Can you work these out from the model? Positions are in its coordinate system, mm. Face numbers are marked on the shaded views. A direction names the side the tool comes from. Give positions to 0.01 mm unless a question says otherwise; leave off trailing zeros. Loops run counter-clockwise (first coordinate to the right, second up) from the corner with the lowest first, then second, coordinate; pieces in that order, holes last. Notation, with made-up numbers: (-38, 30.25) -> (-3, 30.25) arc R29 cw to (-3, 63.25) -> close; hole circle Ø4 at (32, -11). An arc over 180 degrees is marked (long way). One line per question, with ' | ' between items.
from build123d import *

# Parameters (mm, degrees)
F0_R     = 11.5
F1_DEPTH = 1.5
F3_R     = 6.1353913868
F3_R_2   = 4
F4_DEPTH = 0.762
F2_R     = 4
F5_DEPTH = 3


# Not quite as in the source:
# - a fillet or chamfer that OpenCascade refuses, or shapes differently, is made with other operations: its cross-section is extruded or revolved along the edge and cut away or added


with BuildPart() as f1:
    # F0 (on Top) → F1 (new body)
    with BuildSketch(Plane.XY):
        Circle(F0_R)
    extrude(amount=F1_DEPTH)

    # F3 (on face) → F4 (join)
    with BuildSketch(Plane.XY.offset(1.5)):
        Circle(F3_R)
        Circle(F3_R_2, mode=Mode.SUBTRACT)
    extrude(amount=F4_DEPTH)

    # F2 (on face) → F5 (join)
    with BuildSketch(Plane.XY.offset(1.5)):
        Circle(F2_R)
    extrude(amount=F5_DEPTH)

    # F6: fillet of radius 3.6792614691 on 1 edges, made by hand

    # F6_s1 → F6_t2 (revolve, cut)
    with BuildSketch(Plane.XZ):
        with BuildLine():
            ThreePointArc((11.5, 1.5), (10.1967383184, 0.396348303), (8.5355802579, 0))
            Line((8.5355802579, 0), (11.5, 0))
            Line((11.5, 0), (11.5, 1.5))
        make_face()
    revolve(axis=Axis((0, 0, 0), (0, 0, 1)), mode=Mode.SUBTRACT)


solid = f1.part
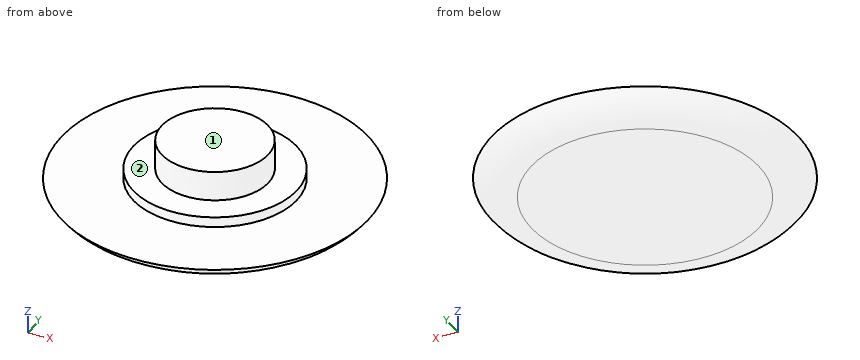
Q1. If we section it at D-D (z = 1.1): Write out the boundary of the cut face in (x, y).
Entries:
outline: circle Ø22.32 at (0, 0)
Q2. If we section it at C-C (z = 3.9): Write out the boundary of the cut face in (x, y), plus the area to 3 significant figures.
Entries:
outline: circle Ø8 at (0, 0) | area: 50.3 mm²
Q3. If we section it at A-A (y = 0): Write out the boundary of the cut face in (x, z), plus the area to 3 significant figures.
Entries:
outline: (-11.5, 1.5) arc R3.68 ccw to (-8.54, 0) -> (8.54, 0) arc R3.68 ccw to (11.5, 1.5) -> (6.14, 1.5) -> (6.14, 2.26) -> (4, 2.26) -> (4, 4.5) -> (-4, 4.5) -> (-4, 2.26) -> (-6.14, 2.26) -> (-6.14, 1.5) -> close | area: 59.1 mm²
Q4. On a 3-axis mill with a long thin cutter (end or side, diameter ignored), from which of +Z, -Z, +X, -X, +Y, -Y can I reach the whole of each face in a straight line? I mean the marked faces 1 and 2. Say none if no direction works.
Entries:
face 1: +Z, +X, -X, +Y, -Y | face 2: +Z
Q5. If I drill on probe 1 along Z at (x, y) = (0.5, 5.25); probe 2 along Y at (x, z) = (0, 2.4); probe 3 along Z at (x, y) = (1, -6.75), over which ranges is the centre line in solid material (lowest first)? Write a range as from..to.
Entries:
probe 1: 0..2.26 | probe 2: -4..4 | probe 3: 0..1.5
